Autodesk Inventor part; units mm, degrees
ref_plane "YZ Plane" through (0, 0, 0) normal (1, 0, 0) x (0, 1, 0)
ref_plane "XZ Plane" through (0, 0, 0) normal (0, 1, 0) x (-1, 0, 0)
ref_plane "XY Plane" through (0, 0, 0) normal (0, 0, 1) x (1, 0, 0)
sketch "Sketch1" plane through (0, 0, 0) normal (0, 1, 0) x (-1, 0, 0)
  line L0 (0, 0) -> (-69.85, 0)
  line L1 (-69.85, 0) -> (-69.85, -946.15)
  line L2 (-69.85, -946.15) -> (0, -946.15)
  line L3 (0, -946.15) -> (0, 0)
  dimension "d0" = 946.15
  dimension "d1" = 69.85
extrude "Extrusion1" add sketch "Sketch1" along normal blind 127
sketch "Sketch2" plane through (69.85, 0, 0) normal (1, 0, 0) x (0, 0, -1)
  line L0 (0, 127) -> (69.85, 127)
  line L1 (69.85, 127) -> (69.85, 0)
  line L2 (69.85, 0) -> (0, 0)
  line L3 (0, 0) -> (0, 127)
  point P0 (946.15, 127)
  dimension "d4" = 69.85
extrude "Extrusion2" add sketch "Sketch2" along normal blind 152.4
sketch "Sketch3" plane through (69.85, 0, -946.15) normal (1, 0, 0) x (0, 0, -1)
  line L0 (0, 0) -> (0, 127)
  line L1 (-876.3, 127) -> (0, 127)
  line L2 (0, 0) -> (-69.85, 0)
  line L3 (-69.85, 0) -> (-69.85, 127)
  line L4 (-69.85, 127) -> (0, 127)
  line L5 (0, 127) -> (0, 0)
  point P0 (-946.15, 0)
  dimension "d8" = 69.85
extrude "Extrusion3" add sketch "Sketch3" along normal blind 342.9
fillet "Fillet1" radius 25.4 1 edges at (222.25, 127, -34.925)
fillet "Fillet2" radius 25.4 1 edges at (412.75, 127, -911.225)
fillet "Fillet6" radius 25.4 3 edges at (193.675, 127, -946.15) (405.3105, 119.5605, -946.15) (412.75, 50.8, -946.15)
fillet "Fillet7" radius 25.4 3 edges at (0, 127, -460.375) (0, 119.5605, -938.7105) (0, 50.8, -946.15)
fillet "Fillet8" radius 25.4 5 edges at (214.8105, 119.5605, 0) (222.25, 50.8, 0) (7.4395, 119.5605, 0) (0, 50.8, 0) (111.125, 127, 0)
sketch "Sketch4" plane through (412.75, 0, -946.15) normal (1, 0, 0) x (0, 0, -1)
  line L0 (-25.4, 101.6) -> (-25.4, 0)
  line L1 (-69.85, 101.6) -> (-25.4, 101.6)
  line L2 (-25.4, 0) -> (-69.85, 0)
  line L3 (-69.85, 0) -> (-69.85, 101.6)
  line L4 (-69.85, 101.6) -> (-25.4, 101.6)
  line L5 (-25.4, 101.6) -> (-25.4, 0)
  point P0 (-946.15, 0)
extrude "Extrusion4" add sketch "Sketch4" along normal blind 12.7
sketch "Sketch5" plane through (425.45, 0, -946.15) normal (1, 0, 0) x (0, 0, -1)
  line L0 (-69.85, 101.6) -> (-69.85, 0)
  line L1 (-69.85, 101.6) -> (-25.4, 101.6)
  line L2 (-25.4, 101.6) -> (-25.4, 0)
  line L3 (-25.4, 0) -> (-69.85, 0)
  line L4 (-69.85, 0) -> (-69.85, 101.6)
  point P0 (-946.15, 0)
extrude "Extrusion5" cut sketch "Sketch5" against normal blind 12.7
fillet "Fillet9" radius 25.4 19 edges at (214.8105, 0, -7.4395) (222.25, 0, -47.625) (7.4395, 0, -7.4395) (0, 0, -473.075) (7.4395, 0, -938.7105) (206.375, 0, -946.15) (405.3105, 0, -938.7105) (412.75, 0, -898.525) (111.125, 0, 0) (146.05, 0, -69.85) (69.85, 0, -473.075) (241.3, 0, -876.3) (405.3105, 119.5605, -876.3) (228.6, 127, -876.3) (412.75, 50.8, -876.3) (214.8105, 119.5605, -69.85) (133.35, 127, -69.85) (222.25, 50.8, -69.85) (69.85, 127, -473.075)
equation "\"BendRadius\" = Thickness"
equation "\"BendReliefWidth\" = Thickness"
equation "\"BendReliefDepth\" = 0.5 * Thickness"
equation "\"CornerReliefSize\" = 4 * Thickness"
equation "\"MinimumRemnant\" = 2 * Thickness"
equation "\"TransitionRadius\" = BendRadius"
equation "\"JacobiRadiusSize\" = BendRadius"
equation "\"GapSize\" = Thickness"
properties part number "Bumpers_2020"
Verification items for the finished model (mm, model axes). A direction names the side the tool comes from. Round coordinates to 2 decimals unless told otherwise and drop trailing zeros. Loops run counter-clockwise (first coordinate to the right, second up) from the corner with the lowest first, then second, coordinate; pieces in that order, holes last. Notation, with made-up numbers: (27.25, 88) - (32.25, 88) arc R7 cw to (32.25, 92) - close; hole circle Ø7 at (53, 20). An arc over 180 degrees is marked (long way). Answer in a Markdown table with one row per item. Add a question column.
Q1. Section check B-B on y = 63.5. Enter the section's corners in (x, z).
Q2. Section check A-A on x = 88. Enter the section's corners in (y, z).
Q3. Release check for a two-part mould opening along Z. For faces 5 (the face through (0, 63, -479)), 6 (the face through (218.3, 119.76, -883.94)), 7 (the face through (7.64, 64.03, -938.91)) record: pulls with the +Z half, pulls with the -Z half, needs draft (parallel to the pull), parting line crosses it, or undercut.
Q4. Section check C-C on x = 338.5. Enter the section's corners in (y, z), plus the area to 3 significant figures.
Q5. Gauge pin test, flat ends, axial feed: pin 1 (3 mm diameter, centred on y = 20, z = -421.5, fed in from -X); pin 2 (6 mm diameter, centred on x = 76.5, y = 62, fed in from +Z); pin 3 (15 mm diameter, centred on y = 47.5, z = -36.5, fed in from +X). Record the tip position at first contact, or that the pin passes through.
Q6. Section check D-D on z = -342.5. Enter the section's corners in (x, y).
Q7. Material ranges on line 1 (Z direction, x = 348.5, y = 65); line 2 (Z direction, x = 78, y = 117.5); line 3 (Z direction, x = 170.5, y = 99.5), recorded low to high.
Q8. Tool access check on faces 1 (the face through (62.61, 7.64, -479.08)), 2 (the face through (222.25, 64, -35)), 3 (the face through (214.61, 119.76, -35.06)), 4 (the face through (214.61, 62.97, -62.61)). Record the directions out of +Z, -Z, +X, -X, +Y, -Y that give a thin tool (end or side, any length) a straight path to the whole face; none if there is none.
Found:
| question | item | result |
|---|---|---|
| 1 | outline | (0, -920.75) arc R25.4 ccw to (25.4, -946.15) - (387.35, -946.15) arc R25.4 ccw to (412.75, -920.75) - (412.75, -901.7) arc R25.4 ccw to (387.35, -876.3) - (69.85, -876.3) - (69.85, -69.85) - (196.85, -69.85) arc R25.4 ccw to (222.25, -44.45) - (222.25, -25.4) arc R25.4 ccw to (196.85, 0) - (25.4, 0) arc R25.4 ccw to (0, -25.4) - close |
| 2 | outline | (0, -920.75) arc R25.4 ccw to (25.4, -946.15) - (101.6, -946.15) arc R25.4 ccw to (127, -920.75) - (127, -901.7) arc R25.4 ccw to (101.6, -876.3) - (25.4, -876.3) arc R25.4 ccw to (0, -901.7) - close; (0, -44.45) arc R25.4 ccw to (25.4, -69.85) - (101.6, -69.85) arc R25.4 ccw to (127, -44.45) - (127, -25.4) arc R25.4 ccw to (101.6, 0) - (25.4, 0) arc R25.4 ccw to (0, -25.4) - close |
| 3 | face 5 | needs draft |
| 3 | face 6 | undercut |
| 3 | face 7 | pulls with the -Z half |
| 4 | outline | (0, -920.75) arc R25.4 ccw to (25.4, -946.15) - (101.6, -946.15) arc R25.4 ccw to (127, -920.75) - (127, -901.7) arc R25.4 ccw to (101.6, -876.3) - (25.4, -876.3) arc R25.4 ccw to (0, -901.7) - close |
| 4 | area | 8,320 mm² |
| 5 | pin 1 | stops at x = 0.3 |
| 5 | pin 2 | stops at z = 0 |
| 5 | pin 3 | stops at x = 222.25 |
| 6 | outline | (0, 25.4) arc R25.4 ccw to (25.4, 0) - (44.45, 0) arc R25.4 ccw to (69.85, 25.4) - (69.85, 101.6) arc R25.4 ccw to (44.45, 127) - (25.4, 127) arc R25.4 ccw to (0, 101.6) - close |
| 7 | line 1 | z = -946.15 to -876.3 |
| 7 | line 2 | z = -940.56 to -881.89, -64.26 to -5.59 |
| 7 | line 3 | z = -946.15 to -876.3, -69.85 to 0 |
| 8 | face 1 | +X, -Y |
| 8 | face 2 | +Z, +X, +Y, -Y |
| 8 | face 3 | +Z, +X, +Y |
| 8 | face 4 | +X, +Y, -Y |
